The listing builds one solid part. Answer for the finished solid, in the listing's coordinates (mm). A direction names the side the tool comes from. Round coordinates to 2 decimals unless told otherwise and drop trailing zeros. Loops run counter-clockwise (first coordinate to the right, second up) from the corner with the lowest first, then second, coordinate; pieces in that order, holes last. Notation, with made-up numbers: (45.25, 60) -> (88.25, 60) arc R10 ccw to (88.25, 66) -> close; hole circle Ø11 at (57, -6.75). An arc over 180 degrees is marked (long way). One line per question, with ' | ' between items.
from build123d import *

# Parameters (mm, degrees)
BOSS_EXTRUDE1_DEPTH             = 88.5
SKETCH3_W                       = 100
SKETCH3_H                       = 20
BOSS_EXTRUDE2_DEPTH             = 19
CUT_EXTRUDE1_DEPTH              = 16
CUT_EXTRUDE1_DEPTH_BACK         = 92.670605976
SKETCH2_R                       = 1.6
SKETCH4_R                       = 3
CUT_EXTRUDE2_DEPTH              = 19
M3X0_5_TAPPED_HOLE1_D           = 2.5
M3X0_5_TAPPED_HOLE1_DEPTH       = 7.5
M3X0_5_TAPPED_HOLE1_CSINK_D     = 3.05
M3X0_5_TAPPED_HOLE1_CSINK_ANGLE = 90
M3X0_5_TAPPED_HOLE1_TIP         = 0.751075774
SKETCH9_R                       = 3.25
CUT_EXTRUDE3_DEPTH              = 10


with BuildPart() as part:
    # Sketch1 → Boss-Extrude1 (new, symmetric)
    with BuildSketch(Plane(origin=(0, 0, 0), x_dir=(0, 0, -1), z_dir=(1, 0, 0))):
        Polygon((-14.5, 0), (14.5, 0), (14.5, 11), (12.55, 11), (12.55, 2), (-12.55, 2), (-12.55, 11), (-14.5, 11), align=None)
    extrude(amount=BOSS_EXTRUDE1_DEPTH, both=True)

    # Sketch3 → Boss-Extrude2 (add)
    with BuildSketch(Plane.XZ):
        Rectangle(SKETCH3_W, SKETCH3_H)
    extrude(amount=BOSS_EXTRUDE2_DEPTH)

    # Sketch2 → Cut-Extrude1 (cut, two sides: drawn at the far end of the back side and taken through both)
    with BuildSketch(Plane.XZ.offset(-CUT_EXTRUDE1_DEPTH_BACK)):
        with Locations(Location((76, 0, 0), (0, 0, 90))):
            Circle(SKETCH2_R)
        with Locations(Location((31, 0, 0), (0, 0, 270))):
            Circle(SKETCH2_R)
        with Locations(Location((-31, 0, 0), (0, 0, 90))):
            Circle(SKETCH2_R)
        with Locations(Location((-76, 0, 0), (0, 0, 90))):
            Circle(SKETCH2_R)
    extrude(amount=CUT_EXTRUDE1_DEPTH + CUT_EXTRUDE1_DEPTH_BACK, mode=Mode.SUBTRACT)

    # Sketch4 → Cut-Extrude2 (cut)
    with BuildSketch(Plane.XZ.offset(19)):
        with Locations(Location((-31, 0, 0), (0, 0, 270))):
            Circle(SKETCH4_R)
        with Locations(Location((31, 0, 0), (0, 0, 270))):
            Circle(SKETCH4_R)
    extrude(amount=-CUT_EXTRUDE2_DEPTH, mode=Mode.SUBTRACT)

    # M3x0.5 Tapped Hole1
    with Locations(Plane(origin=(0, -19, 0), x_dir=(-1, 0, 0), z_dir=(0, -1, 0))):
        with Locations((-26.5, -6), (26.5, 6), (26.5, -6), (-26.5, 6)):
            CounterSinkHole(M3X0_5_TAPPED_HOLE1_D / 2, M3X0_5_TAPPED_HOLE1_CSINK_D / 2, depth=M3X0_5_TAPPED_HOLE1_DEPTH, counter_sink_angle=M3X0_5_TAPPED_HOLE1_CSINK_ANGLE)
            with Locations((0, 0, -(M3X0_5_TAPPED_HOLE1_DEPTH + M3X0_5_TAPPED_HOLE1_TIP / 2))):  # 118° drill point
                Cone(0, M3X0_5_TAPPED_HOLE1_D / 2, M3X0_5_TAPPED_HOLE1_TIP, mode=Mode.SUBTRACT)

    # Sketch9 → Cut-Extrude3 (cut)
    with BuildSketch(Plane.XZ.offset(19)):
        with Locations((14.158699622, -10.285)):
            Circle(SKETCH9_R)
        with Locations((-14.158699622, -10.285)):
            Circle(SKETCH9_R)
        with Locations((-14.158699622, 10.285)):
            Circle(SKETCH9_R)
        with Locations((14.158699622, 10.285)):
            Circle(SKETCH9_R)
    extrude(amount=-CUT_EXTRUDE3_DEPTH, mode=Mode.SUBTRACT)


solid = part.part
Q1. For faces 1 (the face through (-1, -9, 10)), 2 (the face through (14.091, -14.07, 7.036)), 3 (the face through (-1, -9, -10)), 4 (the face through (-32.3, 0, -1.3)), 5 (the face through (-14, -9, -9)), determine the directions among +Z, -Z, +X, -X, +Y, -Y from which every point of the face is accessible in a straight line to the end or side of a thin tool.
Numbers:
face 1: +Z, +X, -X, -Y | face 2: +Z, -Y | face 3: -Z, +X, -X, -Y | face 4: -Y | face 5: -Z, -Y
Q2. For a pull along Z with two mould halves and no side action, classify faces 6 (the face through (1, 6, 14.5)), 7 (the face through (-50, -9, 0)), 8 (the face through (29.7, 0, -1.3)), 9 (the face through (1, 7, -12.55)) as pulls with the +Z half, pulls with the -Z half, needs draft (parallel to the pull), parting line crosses it, or undercut.
Numbers:
face 6: pulls with the +Z half | face 7: needs draft | face 8: undercut | face 9: undercut
Q3. Find the intervals of material crossed by line 1 (X direction, y = -15.75, z = 6); line 2 (X direction, y = -10.5, z = 0); line 3 (X direction, y = 1.1, z = 0), in increasing order. Write a range as from..to.
Numbers:
line 1: -50..-27.75, -25.25..25.25, 27.75..50 | line 2: -50..-34, -28..28, 34..50 | line 3: -88.5..-77.6, -74.4..-32.6, -29.4..29.4, 32.6..74.4, 77.6..88.5
Q4. A cutting plane is placed at B-B on y = -13.75. Give the vertices of the cut face in (x, z) (3 decimals), plus the area to 3 significant figures.
Numbers:
outline: (-50, -10) -> (-17.396, -10) arc R3.25 cw to (-10.921, -10) -> (10.921, -10) arc R3.25 cw to (17.396, -10) -> (50, -10) -> (50, 10) -> (17.396, 10) arc R3.25 cw to (10.921, 10) -> (-10.921, 10) arc R3.25 cw to (-17.396, 10) -> (-50, 10) -> close; hole circle Ø6 at (-31, 0); hole circle Ø2.5 at (-26.5, -6); hole circle Ø2.5 at (-26.5, 6); hole circle Ø2.5 at (26.5, -6); hole circle Ø2.5 at (26.5, 6); hole circle Ø6 at (31, 0) | area: 1,860 mm^2
Q5. A cutting plane is placed at A-A on x = 31. Give the vertices of the cut face in (y, z).
Numbers:
outline: (-19, -10) -> (0, -10) -> (0, -14.5) -> (11, -14.5) -> (11, -12.55) -> (2, -12.55) -> (2, -1.6) -> (0, -1.6) -> (0, -3) -> (-19, -3) -> close; (-19, 3) -> (0, 3) -> (0, 1.6) -> (2, 1.6) -> (2, 12.55) -> (11, 12.55) -> (11, 14.5) -> (0, 14.5) -> (0, 10) -> (-19, 10) -> close
Q6. A cutting plane is placed at D-D on x = 76. Give the vertices of the cut face in (y, z), plus the area to 3 significant figures.
Numbers:
outline: (0, -14.5) -> (11, -14.5) -> (11, -12.55) -> (2, -12.55) -> (2, -1.6) -> (0, -1.6) -> close; (0, 1.6) -> (2, 1.6) -> (2, 12.55) -> (11, 12.55) -> (11, 14.5) -> (0, 14.5) -> close | area: 86.7 mm^2
Q7. Given pin 1 Ø5 at (x, z) = (31, 0) entering from +Y; pin 2 Ø3 at (x, y) = (-33.5, -7) entering from +Z; pin 3 Ø1 at (x, z) = (51, 10.5) entering from -Y; pin 4 Ø3 at (x, y) = (50, -0.5) entering from +Z, each flat-ended and moving along its own axis, determine where each tip first touches the part or whether it passes through.
Numbers:
pin 1: y = 2 | pin 2: z = 10 | pin 3: y = 0 | pin 4: z = 14.5
Q8. A cutting plane is placed at C-C on y = 7. Give the vertices of the cut face in (x, z), plus the area to 3 significant figures.
Numbers:
outline: (-88.5, -14.5) -> (88.5, -14.5) -> (88.5, -12.55) -> (-88.5, -12.55) -> close; (-88.5, 12.55) -> (88.5, 12.55) -> (88.5, 14.5) -> (-88.5, 14.5) -> close | area: 690 mm^2
